Read the model definition and answer for the solid it produces. Units are mm, in the model's axes. Coordinates: 2 decimals unless noted, no trailing zeros. Loops run counter-clockwise (first coordinate to the right, second up) from the corner with the lowest first, then second, coordinate; pieces in that order, holes last.
Q1. Section B-B (y = -20) is taken. Give the vertices of the cut face in (x, z), then the cut area to 3 significant figures.
Q2. Section A-A (z = 3.75) is taken. Give the vertices of the cut face in (x, y), then the cut area to 3 significant figures.
Q3. Section C-C (x = 8.25) is taken. Give the vertices of the cut face in (y, z).
Q4. Straight lines are drawn through the part: line 1 (X direction, y = -25, z = 2.75); line 2 (Y direction, x = 4.5, z = -6.75); line 3 (X direction, y = -71.5, z = -5). For each, find the intervals that lie inside material, in ascending order.
Q5. Flat-ended cylindrical pins translate along their axes: P1, Ø1, axis at x = -2.5, y = -37.5, coming from the +Z side; P2, Ø2, axis at y = -28, z = 2, coming from the -X side; P3, Ø6, axis at y = -40, z = -4, coming from the -X side. Find the tip coordinate at first contact, or state that the pin passes through.
Q6. Section D-D (y = -66) is taken. Give the vertices of the cut face in (x, z), then the cut area to 3 significant figures.
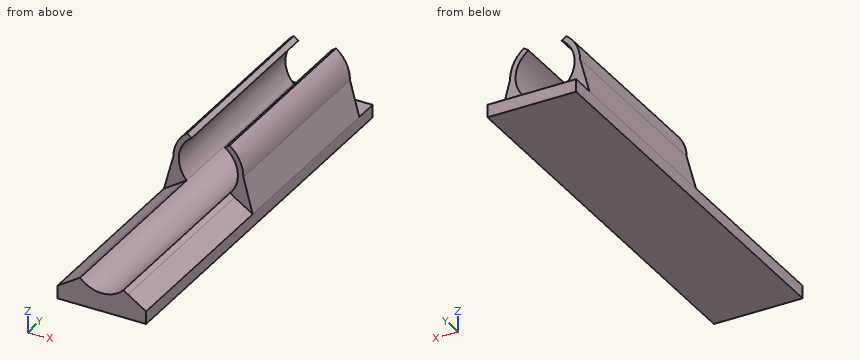
from build123d import *

# Parameters (mm, degrees)
F0_W     = 9.3780029565
F0_H     = 2.6930641449
F1_DEPTH = 80
F2_DEPTH = 40
F3_W     = 18.756005913
F3_H     = 2.6930641449
F4_DEPTH = 5


with BuildPart() as f1:
    # F0 (on Front) → F1 (new body)
    with BuildSketch(Plane.XZ):
        with BuildLine():
            ThreePointArc((4.5775509482, -4.2554115332), (0, -6.25), (-4.5775509482, -4.2554115332))
            Line((-4.5775509482, -4.2554115332), (-5.5563090648, -4.8979718597))
            ThreePointArc((-5.5563090648, -4.8979718597), (-3.0482564998, -6.7506170883), (0, -7.4069358551))
            ThreePointArc((0, -7.4069358551), (3.0482564998, -6.7506170883), (5.5563090648, -4.8979718597))
            Line((5.5563090648, -4.8979718597), (4.5775509482, -4.2554115332))
        make_face()
        with BuildLine():
            Line((9.3780029565, -7.4069358551), (5.5563090648, -4.8979718597))
            ThreePointArc((5.5563090648, -4.8979718597), (3.0482564998, -6.7506170883), (0, -7.4069358551))
            Line((0, -7.4069358551), (9.3780029565, -7.4069358551))
        make_face()
        with BuildLine():
            ThreePointArc((0, -7.4069358551), (-3.0482564998, -6.7506170883), (-5.5563090648, -4.8979718597))
            Line((-5.5563090648, -4.8979718597), (-9.3780029565, -7.4069358551))
            Line((-9.3780029565, -7.4069358551), (0, -7.4069358551))
        make_face()
        with Locations((-4.6890014783, -8.7534679275)):
            Rectangle(F0_W, F0_H)
        with Locations((4.6890014783, -8.7534679275)):
            Rectangle(F0_W, F0_H)
    extrude(amount=F1_DEPTH)

    # F0 (on Front) → F2 (join)
    with BuildSketch(Plane.XZ):
        with BuildLine():
            Line((-9.3780029565, -7.4069358551), (-5.5563090648, -4.8979718597))
            ThreePointArc((-5.5563090648, -4.8979718597), (-6.9288499621, -2.6179642785), (-7.4069358551, 0))
            Line((-7.4069358551, 0), (-9.3780029565, -7.4069358551))
        make_face()
        with BuildLine():
            ThreePointArc((-4.5775509482, -4.2554115332), (-6.2096209441, 0.7093008742), (-3.5, 5.1780787943))
            Line((-3.5, 5.1780787943), (-4.4709416805, 5.9053686803))
            ThreePointArc((-4.4709416805, 5.9053686803), (-6.6324458912, 3.2974778636), (-7.4069358551, 0))
            ThreePointArc((-7.4069358551, 0), (-6.9288499621, -2.6179642785), (-5.5563090648, -4.8979718597))
            Line((-5.5563090648, -4.8979718597), (-4.5775509482, -4.2554115332))
        make_face()
        with BuildLine():
            ThreePointArc((3.5, 5.1780787943), (6.2096209441, 0.7093008742), (4.5775509482, -4.2554115332))
            Line((4.5775509482, -4.2554115332), (5.5563090648, -4.8979718597))
            ThreePointArc((5.5563090648, -4.8979718597), (6.9288499621, -2.6179642785), (7.4069358551, 0))
            ThreePointArc((7.4069358551, 0), (6.6324458912, 3.2974778636), (4.4709416805, 5.9053686803))
            Line((4.4709416805, 5.9053686803), (3.5, 5.1780787943))
        make_face()
        with BuildLine():
            ThreePointArc((7.4069358551, 0), (6.9288499621, -2.6179642785), (5.5563090648, -4.8979718597))
            Line((5.5563090648, -4.8979718597), (9.3780029565, -7.4069358551))
            Line((9.3780029565, -7.4069358551), (7.4069358551, 0))
        make_face()
    extrude(amount=F2_DEPTH)

    # F3 (on face) → F4 (join)
    with BuildSketch(Plane(origin=(0, 0, 0), x_dir=(-1, 0, 0), z_dir=(0, 1, 0))):
        with Locations((0, -8.7534679275)):
            Rectangle(F3_W, F3_H)
    extrude(amount=F4_DEPTH)


solid = f1.part
Numbers:
1. outline: (-9.38, -10.1) - (9.38, -10.1) - (9.38, -7.41) - (7.41, 0) arc R7.41 ccw to (4.47, 5.91) - (3.5, 5.18) arc R6.25 cw (long way) to (-3.5, 5.18) - (-4.47, 5.91) arc R7.41 ccw to (-7.41, 0) - (-9.38, -7.41) - close
1. area: 128 mm2
2. outline: (-6.39, -40) - (-5, -40) - (-5, 0) - (-6.39, 0) - close; (5, -40) - (6.39, -40) - (6.39, 0) - (5, 0) - close
2. area: 111 mm2
3. outline: (-80, -10.1) - (5, -10.1) - (5, -7.41) - (0, -7.41) - (0, -3.17) - (-40, -3.17) - (-40, -6.67) - (-80, -6.67) - close
4. line 1: x = -6.88 to -5.61, 5.61 to 6.88
4. line 2: y = -80 to 0
4. line 3: x = -5.71 to -3.75, 3.75 to 5.71
5. P1: stops at z = -5.48
5. P2: stops at x = -7.34
5. P3: stops at x = -9.27
6. outline: (-9.38, -10.1) - (9.38, -10.1) - (9.38, -7.41) - (4.58, -4.26) arc R6.25 cw to (-4.58, -4.26) - (-9.38, -7.41) - close
6. area: 81.9 mm2
